```python
from build123d import *

# Parameters (mm, degrees)
F0_W     = 76.2
F0_H     = 50.8
F1_DEPTH = 12.7
F3_D     = 38.1


with BuildPart() as f1:
    # F0 (on Front) → F1 (new body, symmetric)
    with BuildSketch(Plane.XZ):
        with Locations((38.1, 25.4)):
            Rectangle(F0_W, F0_H)
    extrude(amount=F1_DEPTH, both=True)

    # F3 (through all)
    with Locations(Plane.XZ.offset(12.7)):
        with Locations((38.1, 25.4)):
            Hole(F3_D / 2)


solid = f1.part
```
Check sheet for the modelled part. Datum: model origin and axes. Units: mm. Coordinates: 2 decimals unless noted, no trailing zeros. Loops run counter-clockwise (first coordinate to the right, second up) from the corner with the lowest first, then second, coordinate; pieces in that order, holes last.
1) Release check for a two-part mould opening along X. For faces 1 (the face through (76.2, 0, 25)), 2 (the face through (0, 0, 25)), 3 (the face through (42.23, 0.178, 6.803)), 4 (the face through (38, 0, 50.8)) record: released by +X, released by -X, zero draft, split by the parting line, or undercut.
2) Material ranges on probe 1 along Z at (x, y) = (38.1, 2); probe 2 along X at (y, z) = (3.75, 39); probe 3 along Z at (x, y) = (43, -4.25), recorded low to high.
3) Sectioned sample at A-A (x = 38.1). Record the boundary of the cut face in (y, z).
4) Sectioned sample at C-C (y = -2). Record the boundary of the cut face in (x, z), and give its area (3 significant figures).
5) Sectioned sample at B-B (z = 25.4). Record the boundary of the cut face in (x, y).
6) Gauge pin test, flat end, axial feed: pin 1 (3 mm diameter, centred on x = 32.5, z = 41, fed in from +Y). Record the tip position at first contact, or that the pin passes through.
Check sheet entries:
1. face 1: released by +X
1. face 2: released by -X
1. face 3: undercut
1. face 4: zero draft
2. probe 1: z = 0 to 6.35, 44.45 to 50.8
2. probe 2: x = 0 to 24.76, 51.44 to 76.2
2. probe 3: z = 0 to 6.99, 43.81 to 50.8
3. outline: (-12.7, 0) - (12.7, 0) - (12.7, 6.35) - (-12.7, 6.35) - close; (-12.7, 44.45) - (12.7, 44.45) - (12.7, 50.8) - (-12.7, 50.8) - close
4. outline: (0, 0) - (76.2, 0) - (76.2, 50.8) - (0, 50.8) - close; hole circle Ø38.1 at (38.1, 25.4)
4. area: 2,730 mm2
5. outline: (0, -12.7) - (19.05, -12.7) - (19.05, 12.7) - (0, 12.7) - close; (57.15, -12.7) - (76.2, -12.7) - (76.2, 12.7) - (57.15, 12.7) - close
6. pin 1: passes through
